from build123d import *

# Parameters (mm, degrees)
MODEL_R                 = 16.5
MODEL_R_2               = 3
MODEL_R_3               = 1.5
SALIENTE_EXTRUIR1_DEPTH = 3


with BuildPart() as part:
    # Model → Saliente-Extruir1 (new body)
    with BuildSketch(Plane.XY):
        with Locations((215.747807914, 241.952019993)):
            Circle(MODEL_R)
        with Locations((215.747807914, 241.952019993)):
            Circle(MODEL_R_2, mode=Mode.SUBTRACT)
        with Locations((215.747807914, 232.952019993)):
            Circle(MODEL_R_3, mode=Mode.SUBTRACT)
        with Locations((215.747807914, 250.952019993)):
            Circle(MODEL_R_3, mode=Mode.SUBTRACT)
        with BuildLine():
            Line((223.122807913, 245.202019993), (221.372807913, 245.202019993))
            ThreePointArc((221.372807913, 245.202019993), (220.842477828, 244.982350079), (220.622807913, 244.452019993))
            Line((220.622807913, 244.452019993), (220.622807913, 239.452019993))
            ThreePointArc((220.622807913, 239.452019993), (220.842477828, 238.921689907), (221.372807913, 238.702019993))
            Line((221.372807913, 238.702019993), (223.122807913, 238.702019993))
            ThreePointArc((223.122807913, 238.702019993), (223.653137999, 238.921689907), (223.872807913, 239.452019993))
            Line((223.872807913, 239.452019993), (223.872807913, 244.452019993))
            ThreePointArc((223.872807913, 244.452019993), (223.653137999, 244.982350079), (223.122807913, 245.202019993))
        make_face(mode=Mode.SUBTRACT)
        with BuildLine():
            Line((208.372807913, 245.202019993), (210.122807913, 245.202019993))
            ThreePointArc((210.122807913, 245.202019993), (210.653137999, 244.982350079), (210.872807913, 244.452019993))
            Line((210.872807913, 244.452019993), (210.872807913, 239.452019993))
            ThreePointArc((210.872807913, 239.452019993), (210.653137999, 238.921689907), (210.122807913, 238.702019993))
            Line((210.122807913, 238.702019993), (208.372807913, 238.702019993))
            ThreePointArc((208.372807913, 238.702019993), (207.842477828, 238.921689907), (207.622807913, 239.452019993))
            Line((207.622807913, 239.452019993), (207.622807913, 244.452019993))
            ThreePointArc((207.622807913, 244.452019993), (207.842477828, 244.982350079), (208.372807913, 245.202019993))
        make_face(mode=Mode.SUBTRACT)
    extrude(amount=SALIENTE_EXTRUIR1_DEPTH)


solid = part.part
Here's how the part is built. I have some questions about the finished solid (model axes, mm). A direction names the side the tool comes from. Coordinates: 2 decimals unless noted, no trailing zeros. Order: outer loops, then holes, each group sorted by start corner. A loop starts at its lowest first (then second) coordinate and runs counter-clockwise, first axis right, second up.
Item 1: If we section it at C-C on z = 2.6: List the corners of the cut face in (x, y) for me, plus the area to 3 significant figures.
Result sheet:
outline: circle Ø33 at (215.75, 241.95); hole (207.62, 239.45) arc R0.75 ccw to (208.37, 238.7) - (210.12, 238.7) arc R0.75 ccw to (210.87, 239.45) - (210.87, 244.45) arc R0.75 ccw to (210.12, 245.2) - (208.37, 245.2) arc R0.75 ccw to (207.62, 244.45) - close; hole circle Ø6 at (215.75, 241.95); hole circle Ø3 at (215.75, 232.95); hole circle Ø3 at (215.75, 250.95); hole (220.62, 239.45) arc R0.75 ccw to (221.37, 238.7) - (223.12, 238.7) arc R0.75 ccw to (223.87, 239.45) - (223.87, 244.45) arc R0.75 ccw to (223.12, 245.2) - (221.37, 245.2) arc R0.75 ccw to (220.62, 244.45) - close
area: 772 mm2
Item 2: If we section it at D-D on y = 250.5: List the corners of the cut face in (x, z) for me, plus the area to 3 significant figures.
Result sheet:
outline: (201.63, 0) - (214.32, 0) - (214.32, 3) - (201.63, 3) - close; (217.18, 0) - (229.86, 0) - (229.86, 3) - (217.18, 3) - close
area: 76.1 mm2
Item 3: If we section it at A-A on y = 243: List the corners of the cut face in (x, z) for me.
Result sheet:
outline: (199.28, 0) - (207.62, 0) - (207.62, 3) - (199.28, 3) - close; (210.87, 0) - (212.94, 0) - (212.94, 3) - (210.87, 3) - close; (218.56, 0) - (220.62, 0) - (220.62, 3) - (218.56, 3) - close; (223.87, 0) - (232.21, 0) - (232.21, 3) - (223.87, 3) - close
Item 4: If we section it at B-B on x = 216: List the corners of the cut face in (y, z) for me, plus the area to 3 significant figures.
Result sheet:
outline: (225.45, 0) - (231.47, 0) - (231.47, 3) - (225.45, 3) - close; (234.43, 0) - (238.96, 0) - (238.96, 3) - (234.43, 3) - close; (244.94, 0) - (249.47, 0) - (249.47, 3) - (244.94, 3) - close; (252.43, 0) - (258.45, 0) - (258.45, 3) - (252.43, 3) - close
area: 63.3 mm2
Item 5: If we mould it in two halves opening along Y, with no side actions, what happens to faces 3 (the face through (215.5, 238.5, 0)), 4 (the face through (213.6, 258.31, 1.48)), 5 (the face through (209, 245.202, 1)), 6 (the face through (215.097, 239.023, 1.479))? For each: +Y half, -Y half, draft (parallel to the pull), parting line (faces both ways), or undercut.
Result sheet:
face 3: draft
face 4: parting line
face 5: undercut
face 6: undercut
Item 6: I need wall thicknesses on line 1 (Y direction, x = 217, z = 0.6); line 2 (X direction, y = 242.5, z = 1.15); line 3 (Y direction, x = 216, z = 2.2). Which ranges of each line are inside material? Lowest first, please.
Result sheet:
line 1: y = 225.5 to 232.13, 233.78 to 239.23, 244.68 to 250.13, 251.78 to 258.4
line 2: x = 199.26 to 207.62, 210.87 to 212.8, 218.7 to 220.62, 223.87 to 232.24
line 3: y = 225.45 to 231.47, 234.43 to 238.96, 244.94 to 249.47, 252.43 to 258.45
Item 7: For P1, Ø0.9, axis at x = 209.5, z = 2, coming from the +Y side; P2, Ø1.5, axis at y = 243, z = 1, coming from the -X side, each with a flat end and sliding along its axis, tell me the tip position at first contact or that it passes through.
Result sheet:
P1: stops at y = 257.4
P2: stops at x = 199.25
Item 8: For faces 1 (the face through (215.5, 238.5, 3)), 2 (the face through (223.873, 242, 1)), which set-ups out of +Z, -Z, +X, -X, +Y, -Y let a thin tool reach every point of the face, with its end or its side?
Result sheet:
face 1: +Z, +X, -X, +Y, -Y
face 2: +Z, -Z
